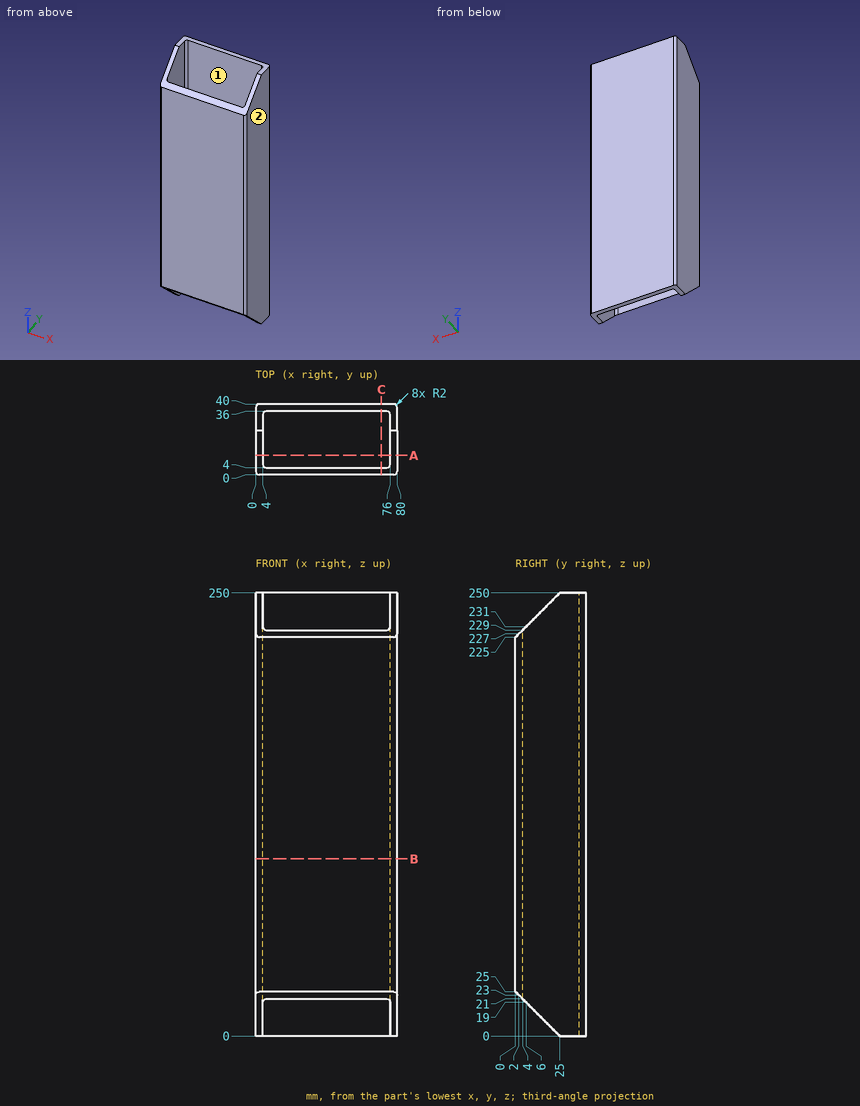
Check sheet for the drawn part. Datum: minimum x, y, z corner. Units: mm. A direction names the side the tool comes from. Round coordinates to 2 decimals unless told otherwise and drop trailing zeros. Order: outer loops, then holes, each group sorted by start corner. A loop starts at its lowest first (then second) coordinate and runs counter-clockwise, first axis right, second up. Notation, with made-up numbers: (40.25, 79.5) -> (97.25, 79.5) arc R27 ccw to (97.25, 109.5) -> close; hole circle Ø8 at (76.25, 67.5). An arc over 180 degrees is marked (long way). Put each result on its own line as item: value. Start each with the question number.
(1) Section check A-A (y = 11). Enter the section's corners in (x, z).
(2) Section check C-C (x = 71). Enter the section's corners in (y, z).
(3) Material ranges on line 1 along X through (y, z) = (33.5, 108.5); line 2 along Y through (x, z) = (65.5, 145); line 3 along Z through (x, y) = (19, 3.5), recorded low to high.
(4) Section check B-B (z = 100). Enter the section's corners in (x, y), then the cut area to 3 significant figures.
(5) Depth check by flat-ended pin: pin 1 Ø2 at (x, y) = (31, 4.5) entering from -Z. Enter the tip coordinate at first touch or a pass-through.
(6) Tool access check on the marked faces 1 and 2. Record the directions out of +Z, -Z, +X, -X, +Y, -Y that give a thin tool (end or side, any length) a straight path to the whole face; none if there is none.
Completed:
1. outline: (0, 14) -> (4, 14) -> (4, 236) -> (0, 236) -> close; (76, 14) -> (80, 14) -> (80, 236) -> (76, 236) -> close
2. outline: (0, 25) -> (4, 21) -> (4, 229) -> (0, 225) -> close; (36, 0) -> (40, 0) -> (40, 250) -> (36, 250) -> close
3. line 1: x = 0 to 4, 76 to 80
3. line 2: y = 0 to 4, 36 to 40
3. line 3: z = 21.5 to 228.5
4. outline: (0, 2) arc R2 ccw to (2, 0) -> (78, 0) arc R2 ccw to (80, 2) -> (80, 38) arc R2 ccw to (78, 40) -> (2, 40) arc R2 ccw to (0, 38) -> close; hole (4, 6) arc R2 ccw to (6, 4) -> (74, 4) arc R2 ccw to (76, 6) -> (76, 34) arc R2 ccw to (74, 36) -> (6, 36) arc R2 ccw to (4, 34) -> close
4. area: 896 mm2
5. pin 1: stops at z = 21
6. face 1: +Z, -Z
6. face 2: +Z, -Z, +X, +Y, -Y
